Geometry check sheet. Reference: drawing and pictorial views, mm from the part's lowest x, y, z. A direction names the side the tool comes from. Coordinates: 2 decimals unless noted, no trailing zeros. Order: outer loops, then holes, each group sorted by start corner. A loop starts at its lowest first (then second) coordinate and runs counter-clockwise, first axis right, second up. Notation, with made-up numbers: M 84.5,27.25 L 93.5,27.25 A25 cw 93.5,66.25 Z; hole C -11,12.25 d4. An arc over 180 degrees is marked long. Return JSON: item names as keys, results as strings.
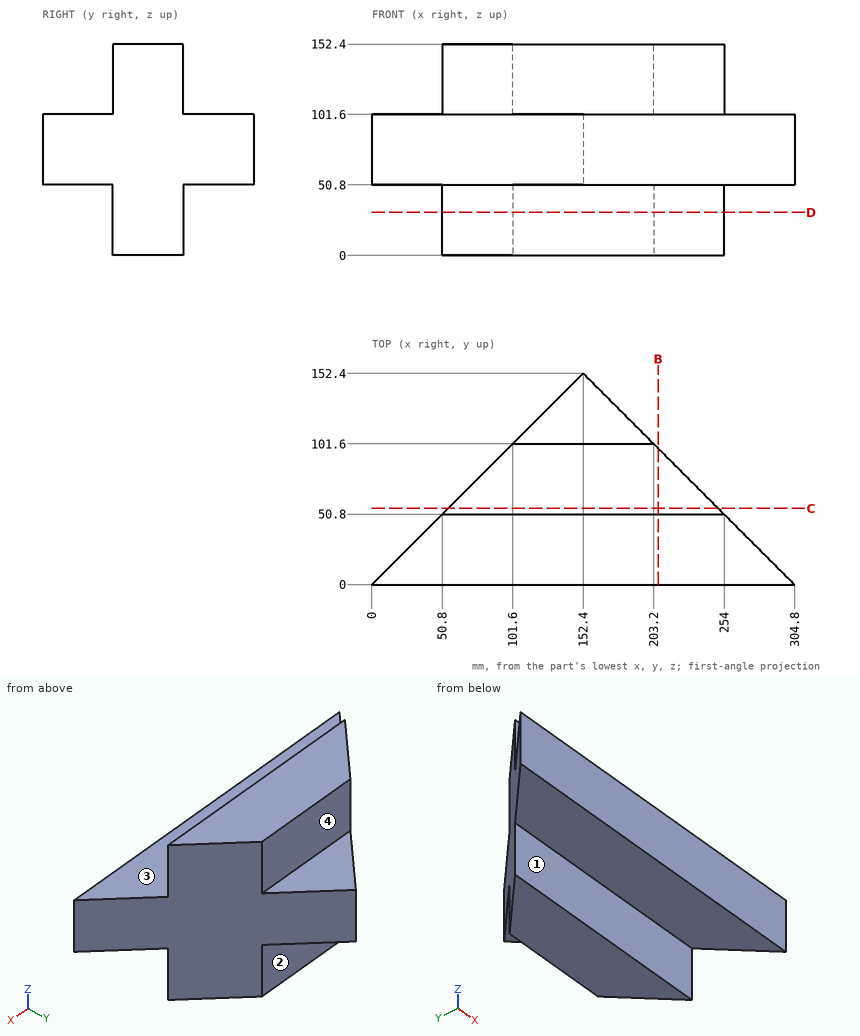
Q1. Tool access check on the marked faces 1, 2, 3 and 4. Record the directions out of +Z, -Z, +X, -X, +Y, -Y that give a thin tool (end or side, any length) a straight path to the whole face; none if there is none.
Values:
{"face 1": "-Z, +X, -X, -Y", "face 2": "-Z, +X, -X, +Y", "face 3": "+Z, +X, -X, -Y", "face 4": "+Z, +X, -X, +Y"}
Q2. Cross-section at D-D, the plane z = 31. Record the boundary of the cut face in (x, y).
Values:
{"outline": "M 50.8,50.8 L 254,50.8 L 203.2,101.6 L 101.6,101.6 Z"}
Q3. Go/stop test with flat-tipped pins: pin 1 (15 mm diameter, centred on x = 157.5, z = 125, fed in from -Y); pin 2 (15 mm diameter, centred on x = 175, z = 130, fed in from +Y); pin 3 (8 mm diameter, centred on x = 91.5, z = 28.5, fed in from +Y). Record where each tip stops, or that it passes through.
Values:
{"pin 1": "y = 50.8", "pin 2": "y = 101.6", "pin 3": "y = 95.5"}
Q4. Cross-section at C-C, the plane y = 55. Record the boundary of the cut face in (x, z), and give its area (3 significant figures).
Values:
{"outline": "M 55,0 L 249.8,0 L 249.8,152.4 L 55,152.4 Z", "area": "29,700 mm^2"}
Q5. Material ranges on line 1 along Y through (x, z) = (185, 45); line 2 along Y through (x, z) = (208.5, 26.5), recorded low to high.
Values:
{"line 1": "50.8 to 101.6", "line 2": "50.8 to 96.3"}
Q6. Cross-section at B-B, the plane x = 206.5. Record the boundary of the cut face in (y, z), and give its area (3 significant figures).
Values:
{"outline": "M 0,50.8 L 50.8,50.8 L 50.8,0 L 98.3,0 L 98.3,152.4 L 50.8,152.4 L 50.8,101.6 L 0,101.6 Z", "area": "9,820 mm^2"}
